```python
from build123d import *

# Parameters (mm, degrees)
SKETCH1_W               = 457.2
SKETCH1_H               = 101.6
BOSS_EXTRUDE1_DEPTH     = 6.35
CUT_EXTRUDE1_DEPTH      = 235.26250767
F_1_4_CLEARANCE_HOLE1_D = 6.7564
MIRROR4_COPY_1_D        = 6.7564
CUT_EXTRUDE2_DEPTH      = 235.26250767
SKETCH7_W               = 317.5
SKETCH7_H               = 101.6
CUT_EXTRUDE3_DEPTH      = 235.26250767
F_1_4_CLEARANCE_HOLE2_D = 6.7564


with BuildPart() as part:
    # Sketch1 → Boss-Extrude1 (new body)
    with BuildSketch(Plane(origin=(0, 0, 0), x_dir=(1, 0, 0), z_dir=(0, 1, 0))):
        Rectangle(SKETCH1_W, SKETCH1_H)
    extrude(amount=BOSS_EXTRUDE1_DEPTH)

    # Sketch2 → Cut-Extrude1 (cut, through all)
    with BuildSketch(Plane(origin=(0, 6.35, 0), x_dir=(1, 0, 0), z_dir=(0, 1, 0))):
        with BuildLine():
            Line((200.025, -41.275), (117.475, -41.275))
            ThreePointArc((117.475, -41.275), (114.3, -38.1), (117.475, -34.925))
            Line((117.475, -34.925), (200.025, -34.925))
            ThreePointArc((200.025, -34.925), (203.2, -38.1), (200.025, -41.275))
        make_face()
    cut_extrude1 = extrude(amount=-CUT_EXTRUDE1_DEPTH, mode=Mode.SUBTRACT)

    # Mirror1: Cut-Extrude1 across plane
    add(cut_extrude1.mirror(Plane.XY), mode=Mode.SUBTRACT)

    # 1/4 Clearance Hole1 (through all)
    with Locations(Plane(origin=(0, 6.35, 0), x_dir=(1, 0, 0), z_dir=(0, 1, 0))):
        with Locations((-215.9, 12.7), (-215.9, 38.1)):
            f_1_4_clearance_hole1 = Hole(F_1_4_CLEARANCE_HOLE1_D / 2)

    # Mirror3: 1/4 Clearance Hole1 across plane
    add(f_1_4_clearance_hole1.mirror(Plane.XY), mode=Mode.SUBTRACT)

    # Mirror4: 1/4 Clearance Hole1 across plane
    add(f_1_4_clearance_hole1.mirror(Plane(origin=(0, 0, 0), x_dir=(0, 0, 1), z_dir=(1, 0, 0))), mode=Mode.SUBTRACT)

    # Mirror4 copy 1 (through all)
    with Locations(Plane(origin=(0, 6.35, 0), x_dir=(-1, 0, 0), z_dir=(0, 1, 0))):
        with Locations((-215.9, 12.7), (-215.9, 38.1)):
            Hole(MIRROR4_COPY_1_D / 2)

    # Sketch6 → Cut-Extrude2 (cut, through all)
    with BuildSketch(Plane(origin=(0, 6.35, 0), x_dir=(1, 0, 0), z_dir=(0, 1, 0))):
        with BuildLine():
            Line((-190.5, 41.275), (-63.5, 41.275))
            ThreePointArc((-63.5, 41.275), (-60.325, 38.1), (-63.5, 34.925))
            Line((-63.5, 34.925), (-190.5, 34.925))
            ThreePointArc((-190.5, 34.925), (-193.675, 38.1), (-190.5, 41.275))
        make_face()
    cut_extrude2 = extrude(amount=-CUT_EXTRUDE2_DEPTH, mode=Mode.SUBTRACT)

    # Mirror5: Cut-Extrude2 across plane
    add(cut_extrude2.mirror(Plane.XY), mode=Mode.SUBTRACT)

    # Sketch7 → Cut-Extrude3 (cut, through all)
    with BuildSketch(Plane(origin=(0, 6.35, 0), x_dir=(1, 0, 0), z_dir=(0, 1, 0))):
        with Locations((-69.85, 0)):
            Rectangle(SKETCH7_W, SKETCH7_H)
    extrude(amount=-CUT_EXTRUDE3_DEPTH, mode=Mode.SUBTRACT)

    # 1/4 Clearance Hole2 (through all)
    with Locations(Plane(origin=(0, 6.35, 0), x_dir=(1, 0, 0), z_dir=(0, 1, 0))):
        with Locations((101.6, 38.1), (101.6, 12.7)):
            f_1_4_clearance_hole2 = Hole(F_1_4_CLEARANCE_HOLE2_D / 2)

    # Mirror8: 1/4 Clearance Hole2 across plane
    add(f_1_4_clearance_hole2.mirror(Plane.XY), mode=Mode.SUBTRACT)


solid = part.part
```
Read the model definition and answer for the solid it produces. Units are mm, in the model's axes. A direction names the side the tool comes from. Round coordinates to 2 decimals unless told otherwise and drop trailing zeros. Write each loop counter-clockwise with the first axis right and the second up, starting at its lowest first coordinate (ties: lowest second). Pieces come first, ordered by that corner, then holes. Notation, with made-up numbers: (83, 26) - (89, 26) arc R18 ccw to (89, 50) - close; hole circle Ø6 at (85, -11.5). An arc over 180 degrees is marked (long way). One line per item, written item: value.
Q1. For a pull along X with two mould halves and no side action, classify faces 3 (the cylindrical face through (114.3, 3.2, 38.2)), 4 (the flat face through (228.6, 3, 1)), 5 (the flat face through (158, 6.35, -1)) as pulls with the +X half, pulls with the -X half, needs draft (parallel to the pull), parting line crosses it, or undercut.
The answers:
face 3: undercut
face 4: pulls with the +X half
face 5: needs draft
Q2. This flat-tipped pin is pushed along its axis until it touches: P1, Ø5.5, axis at x = 215.9, z = -38.1, coming from the -Y side. Where does it stop, or does it pass through?
The answers:
P1: passes through
Q3. Find section B-B (z = 38.1). Determine the outline of the cut face in (x, y), and give its area (3 significant figures).
The answers:
outline: (88.9, 0) - (98.22, 0) - (98.22, 6.35) - (88.9, 6.35) - close; (104.98, 0) - (114.3, 0) - (114.3, 6.35) - (104.98, 6.35) - close; (203.2, 0) - (212.52, 0) - (212.52, 6.35) - (203.2, 6.35) - close; (219.28, 0) - (228.6, 0) - (228.6, 6.35) - (219.28, 6.35) - close
area: 237 mm2
Q4. Find section D-D (x = 101.6). Determine the outline of the cut face in (y, z), and give its area (3 significant figures).
The answers:
outline: (0, -50.8) - (6.35, -50.8) - (6.35, -41.48) - (0, -41.48) - close; (0, -34.72) - (6.35, -34.72) - (6.35, -16.08) - (0, -16.08) - close; (0, -9.32) - (6.35, -9.32) - (6.35, 9.32) - (0, 9.32) - close; (0, 16.08) - (6.35, 16.08) - (6.35, 34.72) - (0, 34.72) - close; (0, 41.48) - (6.35, 41.48) - (6.35, 50.8) - (0, 50.8) - close
area: 474 mm2
Q5. Find section A-A (x = 190). Determine the outline of the cut face in (y, z) (3 decimals).
The answers:
outline: (0, -50.8) - (6.35, -50.8) - (6.35, -41.275) - (0, -41.275) - close; (0, -34.925) - (6.35, -34.925) - (6.35, 34.925) - (0, 34.925) - close; (0, 41.275) - (6.35, 41.275) - (6.35, 50.8) - (0, 50.8) - close
Q6. Find section C-C (z = 12.7). Determine the outline of the cut face in (x, y), and give its area (3 significant figures).
The answers:
outline: (88.9, 0) - (98.22, 0) - (98.22, 6.35) - (88.9, 6.35) - close; (104.98, 0) - (212.52, 0) - (212.52, 6.35) - (104.98, 6.35) - close; (219.28, 0) - (228.6, 0) - (228.6, 6.35) - (219.28, 6.35) - close
area: 801 mm2
Q7. Straight lines are drawn through the part: line 1 (Z direction, x = 101.6, y = 1.5); line 2 (Z direction, x = 125, y = 6) (3 decimals); line 3 (X direction, y = 0.75, z = -14.5). For each, find the intervals that lie inside material, in ascending order. Write a range as from..to.
The answers:
line 1: z = -50.8..-41.48, -34.72..-16.08, -9.32..9.32, 16.08..34.72, 41.48..50.8
line 2: z = -50.8..-41.275, -34.925..34.925, 41.275..50.8
line 3: x = 88.9..98.74, 104.46..213.04, 218.76..228.6
Q8. Which of the six approach directions +Z, -Z, +X, -X, +Y, -Y give full straight-line access (tool end or side, diameter ignored) to faces 1 (the flat face through (158, 0, -1)), 2 (the flat face through (158, 3, -34.925))?
The answers:
face 1: +Z, -Z, +X, -X, -Y
face 2: +Y, -Y
